Can you work these out from the model? Positions are in its coordinate system, mm. A direction names the side the tool comes from. Give positions to 0.01 mm unless a question says otherwise; leave off trailing zeros. Order: outer loops, then holes, each group sorted by start corner. A loop starts at its lowest first (then second) coordinate and runs counter-clockwise, first axis right, second up. Notation, with made-up numbers: (18.5, 56.5) - (59.5, 56.5) arc R21 cw to (59.5, 84.5) - close; hole circle Ø3 at (2.25, -36.5). An arc over 180 degrees is marked (long way). Return JSON: item names as keys, results as strings.
```python
from build123d import *

# Parameters (mm, degrees)
BOSS_EXTRUDE1_DEPTH      = 7
BOSS_EXTRUDE1_DEPTH_BACK = 14.970201
BOSS_EXTRUDE2_START      = -14.970201
SKETCH2_R                = 2
BOSS_EXTRUDE2_DEPTH      = 13.350798149
BOSS_EXTRUDE3_START      = -14.970203
SKETCH3_R                = 1.5
BOSS_EXTRUDE3_DEPTH      = 4.000003


with BuildPart() as part:
    # Sketch1 → Boss-Extrude1 (new, two sides: drawn at the far end of the back side and taken through both)
    with BuildSketch(Plane.XY.offset(-BOSS_EXTRUDE1_DEPTH_BACK)):
        with BuildLine():
            Line((54.999742941, -1.649999966), (5.000257256, -1.649999966))
            ThreePointArc((5.000257256, -1.649999966), (0.297273819, 0.297273819), (-1.649999966, 5.000257256))
            Line((-1.649999966, 5.000257256), (-1.649999966, 54.999742941))
            ThreePointArc((-1.649999966, 54.999742941), (0.297274177, 59.702725823), (5.000257059, 61.649999966))
            Line((5.000257059, 61.649999966), (54.999743139, 61.649999966))
            ThreePointArc((54.999743139, 61.649999966), (59.702725466, 59.702725466), (61.649999966, 54.999743139))
            Line((61.649999966, 54.999743139), (61.649999966, 5.000257059))
            ThreePointArc((61.649999966, 5.000257059), (59.702725823, 0.297274177), (54.999742941, -1.649999966))
        make_face()
        with BuildLine():
            ThreePointArc((5.000039752, 60.249999994), (1.287223653, 58.712776347), (-0.249999994, 54.999960248))
            Line((-0.249999994, 54.999960248), (-0.249999994, 5.000039782))
            ThreePointArc((-0.249999994, 5.000039782), (1.287223296, 1.287223296), (5.000039782, -0.249999994))
            Line((5.000039782, -0.249999994), (54.999960248, -0.249999994))
            ThreePointArc((54.999960248, -0.249999994), (58.712776347, 1.287223653), (60.249999994, 5.000039752))
            Line((60.249999994, 5.000039752), (60.249999994, 54.999960279))
            ThreePointArc((60.249999994, 54.999960279), (58.712775989, 58.712775989), (54.999960279, 60.249999994))
            Line((54.999960279, 60.249999994), (5.000039752, 60.249999994))
        make_face(mode=Mode.SUBTRACT)
    extrude(amount=BOSS_EXTRUDE1_DEPTH + BOSS_EXTRUDE1_DEPTH_BACK)


with BuildPart() as boss_extrude2_tool:
    # Sketch2 → Boss-Extrude2 (new body)
    # profile 1 of 4: a face of its own
    with BuildSketch(Plane.XY.offset(BOSS_EXTRUDE2_START)):
        with BuildLine():
            Line((9.00000016, 54.99999922), (9.00000016, 60.249999994))
            Line((9.00000016, 60.249999994), (5.000039752, 60.249999994))
            add(Edge.make_bspline(
                [(-0.249999994, 54.999960248), (-0.250954892, 58.075921633), (1.924078367, 60.250954892), (5.000039752, 60.249999994)],
                knots=[0, 0, 0, 0, 1, 1, 1, 1], degree=3, weights=[1, 0.804591489, 0.804591489, 1]))
            Line((-0.249999994, 54.999960248), (-0.249999994, 50.99999922))
            Line((-0.249999994, 50.99999922), (5.00000016, 50.99999922))
            ThreePointArc((5.00000016, 50.99999922), (7.828427285, 52.171572095), (9.00000016, 54.99999922))
        make_face()
        with Locations(Location((5.00000016, 54.99999922, 0), (0, 0, 90))):
            Circle(SKETCH2_R, mode=Mode.SUBTRACT)
    # profile 2 of 4: a face of its own
    with BuildSketch(Plane.XY.offset(BOSS_EXTRUDE2_START)):
        with BuildLine():
            Line((50.99999922, 54.99999984), (50.99999922, 60.249999994))
            Line((50.99999922, 60.249999994), (54.999960248, 60.249999994))
            add(Edge.make_bspline(
                [(54.999960248, 60.249999994), (58.075921633, 60.250954892), (60.250954892, 58.075921633), (60.249999994, 54.999960248)],
                knots=[0, 0, 0, 0, 1, 1, 1, 1], degree=3, weights=[1, 0.804591489, 0.804591489, 1]))
            Line((60.249999994, 54.999960248), (60.249999994, 50.99999984))
            Line((60.249999994, 50.99999984), (54.99999922, 50.99999984))
            ThreePointArc((54.99999922, 50.99999984), (52.171572095, 52.171572715), (50.99999922, 54.99999984))
        make_face()
        with Locations(Location((54.99999922, 54.99999984, 0), (0, 0, 90))):
            Circle(SKETCH2_R, mode=Mode.SUBTRACT)
    # profile 3 of 4: a face of its own
    with BuildSketch(Plane.XY.offset(BOSS_EXTRUDE2_START)):
        with BuildLine():
            Line((54.99999984, 9.00000078), (60.249999994, 9.00000078))
            Line((60.249999994, 9.00000078), (60.249999994, 5.000039752))
            add(Edge.make_bspline(
                [(60.249999994, 5.000039752), (60.250954892, 1.924078367), (58.075921633, -0.250954892), (54.999960248, -0.249999994)],
                knots=[0, 0, 0, 0, 1, 1, 1, 1], degree=3, weights=[1, 0.804591489, 0.804591489, 1]))
            Line((54.999960248, -0.249999994), (50.99999984, -0.249999994))
            Line((50.99999984, -0.249999994), (50.99999984, 5.00000078))
            ThreePointArc((50.99999984, 5.00000078), (52.171572715, 7.828427905), (54.99999984, 9.00000078))
        make_face()
        with Locations(Location((54.99999984, 5.00000078, 0), (0, 0, 90))):
            Circle(SKETCH2_R, mode=Mode.SUBTRACT)
    # profile 4 of 4: a face of its own
    with BuildSketch(Plane.XY.offset(BOSS_EXTRUDE2_START)):
        with BuildLine():
            Line((9.00000078, 5.00000016), (9.00000078, -0.249999994))
            Line((9.00000078, -0.249999994), (5.000039752, -0.249999994))
            add(Edge.make_bspline(
                [(5.000039752, -0.249999994), (1.924078367, -0.250954892), (-0.250954892, 1.924078367), (-0.249999994, 5.000039752)],
                knots=[0, 0, 0, 0, 1, 1, 1, 1], degree=3, weights=[1, 0.804591489, 0.804591489, 1]))
            Line((-0.249999994, 5.000039752), (-0.249999994, 9.00000016))
            Line((-0.249999994, 9.00000016), (5.00000078, 9.00000016))
            ThreePointArc((5.00000078, 9.00000016), (7.828427905, 7.828427285), (9.00000078, 5.00000016))
        make_face()
        with Locations(Location((5.00000078, 5.00000016, 0), (0, 0, 90))):
            Circle(SKETCH2_R, mode=Mode.SUBTRACT)
    extrude(amount=BOSS_EXTRUDE2_DEPTH)


with BuildPart() as part_1:
    add(part.part)


with BuildPart() as part_2:
    # Boss-Extrude2: joined with boss_extrude2_tool
    add(part_1.part.fuse(boss_extrude2_tool.part, tol=0.00001))

    # Sketch3 → Boss-Extrude3 (add)
    # profile 1 of 4: a face of its own
    with BuildSketch(Plane.XY.offset(BOSS_EXTRUDE3_START)):
        with BuildLine():
            Line((60.249999994, 23.999999985), (60.249999994, 35.999999985))
            ThreePointArc((60.249999994, 35.999999985), (54.249999994, 29.999999985), (60.249999994, 23.999999985))
        make_face()
        with Locations(Location((57.249999994, 29.999999985, 0), (0, 0, 180))):
            Circle(SKETCH3_R, mode=Mode.SUBTRACT)
    # profile 2 of 4: a face of its own
    with BuildSketch(Plane.XY.offset(BOSS_EXTRUDE3_START)):
        with BuildLine():
            Line((36.000000015, 60.249999994), (24.000000015, 60.249999994))
            ThreePointArc((24.000000015, 60.249999994), (30.000000015, 54.249999994), (36.000000015, 60.249999994))
        make_face()
        with Locations(Location((30.000000015, 57.249999994, 0), (0, 0, 180))):
            Circle(SKETCH3_R, mode=Mode.SUBTRACT)
    # profile 3 of 4: a face of its own
    with BuildSketch(Plane.XY.offset(BOSS_EXTRUDE3_START)):
        with BuildLine():
            Line((23.999999985, -0.249999994), (35.999999985, -0.249999994))
            ThreePointArc((35.999999985, -0.249999994), (29.999999985, 5.750000006), (23.999999985, -0.249999994))
        make_face()
        with Locations(Location((29.999999985, 2.750000006, 0), (0, 0, 180))):
            Circle(SKETCH3_R, mode=Mode.SUBTRACT)
    # profile 4 of 4: a face of its own
    with BuildSketch(Plane.XY.offset(BOSS_EXTRUDE3_START)):
        with BuildLine():
            Line((-0.249999994, 36.000000015), (-0.249999994, 24.000000015))
            ThreePointArc((-0.249999994, 24.000000015), (5.750000006, 30.000000015), (-0.249999994, 36.000000015))
        make_face()
        with Locations(Location((2.750000006, 30.000000015, 0), (0, 0, 180))):
            Circle(SKETCH3_R, mode=Mode.SUBTRACT)
    extrude(amount=BOSS_EXTRUDE3_DEPTH)


solid = part_2.part
```
1. Suppose I cut it at B-B (y = 50). List the corners of the cut face in (x, z) for me, plus the area to 3 significant figures.
Checks:
{"outline": "(-1.65, -14.97) - (-0.25, -14.97) - (-0.25, 7) - (-1.65, 7) - close; (60.25, -14.97) - (61.65, -14.97) - (61.65, 7) - (60.25, 7) - close", "area": "61.5 mm^2"}
2. Thinking about a two-plate mould opening in Y: for faces 1 (the face through (61, 32, -14.97)), 2 (the face through (1.247, 1.328, 2.63)), 3 (the face through (30, 61.65, -4)), which applies, +Y half, -Y half, draft (parallel to the pull), parting line (faces both ways), or undercut?
Checks:
{"face 1": "draft", "face 2": "undercut", "face 3": "+Y half"}
3. For pin 1 Ø1 at (x, y) = (53, 10) entering from +Z; pin 2 Ø3 at (x, y) = (6, 58) entering from +Z; pin 3 Ø4 at (x, z) = (3, -5.5) entering from -Y; pin 4 Ø5 at (x, y) = (28, 57.5) entering from +Z, each with a flat end and sliding along its axis, tell me the tip position at first contact or that it passes through.
Checks:
{"pin 1": "through", "pin 2": "z = -1.62", "pin 3": "y = -1.65", "pin 4": "z = -10.97"}
4. Suppose I cut it at A-A (x = 30). State how many separate pieces and enclosed holes the cut face has, plus the area to 3 significant figures.
Checks:
{"separate pieces": "4", "enclosed holes": "0", "area": "85.5 mm^2"}
5. On a 3-axis mill with a long thin cutter (end or side, diameter ignored), from which of +Z, -Z, +X, -X, +Y, -Y can I reach the whole of each face in a straight line? I mean faces 4 (the face through (30, 59, -10.97)), 5 (the face through (5.75, 29.87, -13)). Say none if no direction works.
Checks:
{"face 4": "+Z", "face 5": "+Z, -Z"}
6. Suppose I cut it at C-C (z = -5). List the corners of the cut face in (x, y) for me.
Checks:
{"outline": "(-1.65, 5) arc R6.65 ccw to (5, -1.65) - (55, -1.65) arc R6.65 ccw to (61.65, 5) - (61.65, 55) arc R6.65 ccw to (55, 61.65) - (5, 61.65) arc R6.65 ccw to (-1.65, 55) - close; hole (-0.25, 9) - (5, 9) arc R4 cw to (9, 5) - (9, -0.25) - (51, -0.25) - (51, 5) arc R4 cw to (55, 9) - (60.25, 9) - (60.25, 51) - (55, 51) arc R4 cw to (51, 55) - (51, 60.25) - (9, 60.25) - (9, 55) arc R4 cw to (5, 51) - (-0.25, 51) - close; hole circle Ø4 at (5, 5); hole circle Ø4 at (5, 55); hole circle Ø4 at (55, 5); hole circle Ø4 at (55, 55)"}
7. If I drill on L1, parallel to Y at x = 55, z = -5; L2, parallel to Y at x = 28.5, z = 4.75, over which ranges is the centre line in solid material (lowest first)? Write a range as [from, to].
Checks:
{"L1": "[-1.65, 3], [7, 9], [51, 53], [57, 61.65]", "L2": "[-1.65, -0.25], [60.25, 61.65]"}
